Part print with two shaded views. Sizes in mm from the minimum x, y, z corner. Round coordinates to 2 decimals unless told otherwise and drop trailing zeros. Loops run counter-clockwise (first coordinate to the right, second up) from the corner with the lowest first, then second, coordinate; pieces in that order, holes last. Notation, with made-up numbers: M 34,40.5 L 51,40.5 A7 cw 51,47.5 Z; hole C 70.5,-3 d3. An arc over 180 degrees is marked long. Answer as CSV lines item,"result". Start each with the question number.
Item 1: Band-saw the part on D-D (y = 2.5). Give the cut face in (x, z), and give its area (3 significant figures).
Item 2: Band-saw the part on C-C (z = 106). Give the cut face in (x, y).
Item 3: Wall check: line 1 (Z direction, x = 57.5, y = 6.75); line 2 (X direction, y = 10, z = 64.5). Give the ranges that are in metal, low to high.
Item 4: Drop flat-ended pins along their axis: pin 1 Ø1.9 at (x, z) = (24, 9.5) entering from +Y; pin 2 Ø4 at (y, z) = (4.5, 23) entering from -X. Give the stop position or say it passes through.
Item 5: Band-saw the part on A-A (y = 11). Give the cut face in (x, z), and give its area (3 significant figures).
Item 6: Band-saw the part on B-B (x = 39). Give the cut face in (y, z).
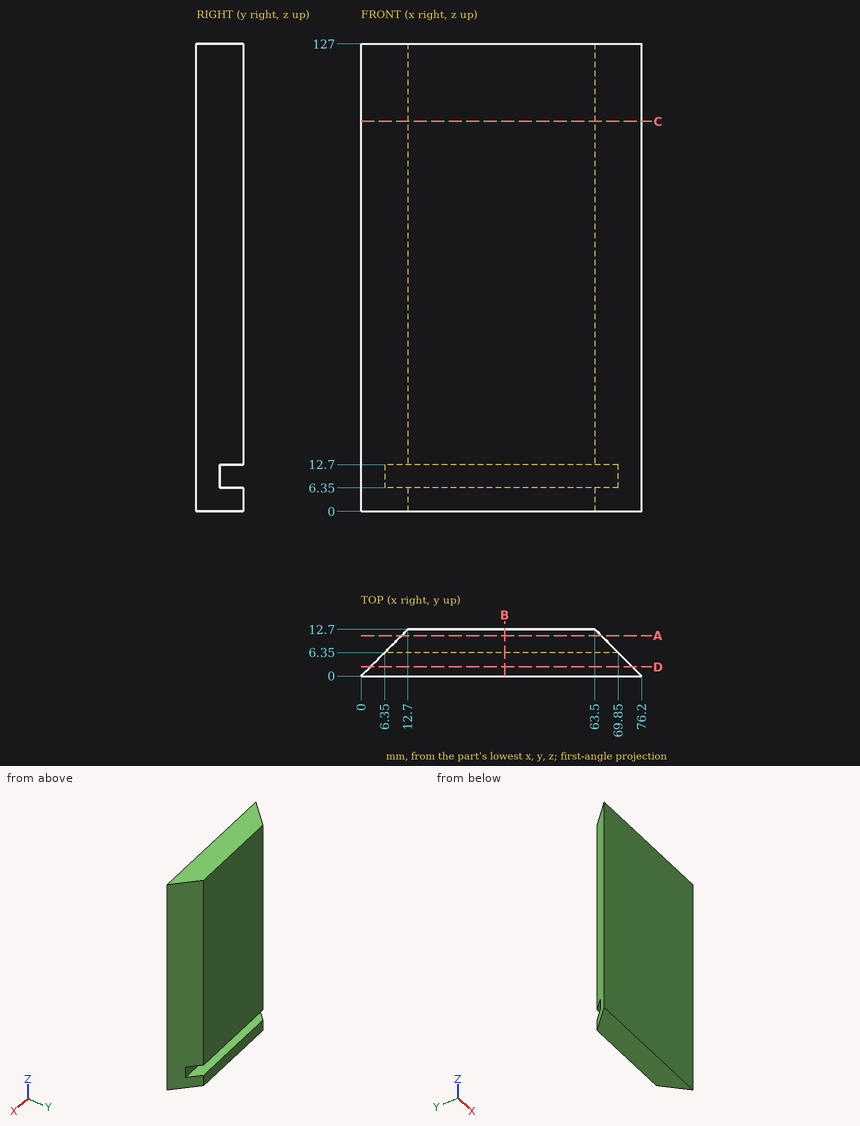
Answer block:
1,outline,"M 2.5,0 L 73.7,0 L 73.7,127 L 2.5,127 Z"
1,area,"9,040 mm^2"
2,outline,"M 0,0 L 76.2,0 L 63.5,12.7 L 12.7,12.7 Z"
3,line 1,"z = 0 to 6.35, 12.7 to 127"
3,line 2,"x = 10 to 66.2"
4,pin 1,"stops at y = 6.35"
4,pin 2,"stops at x = 2.5"
5,outline,"M 11,0 L 65.2,0 L 65.2,6.35 L 11,6.35 Z; M 11,12.7 L 65.2,12.7 L 65.2,127 L 11,127 Z"
5,area,"6,540 mm^2"
6,outline,"M 0,0 L 12.7,0 L 12.7,6.35 L 6.35,6.35 L 6.35,12.7 L 12.7,12.7 L 12.7,127 L 0,127 Z"
